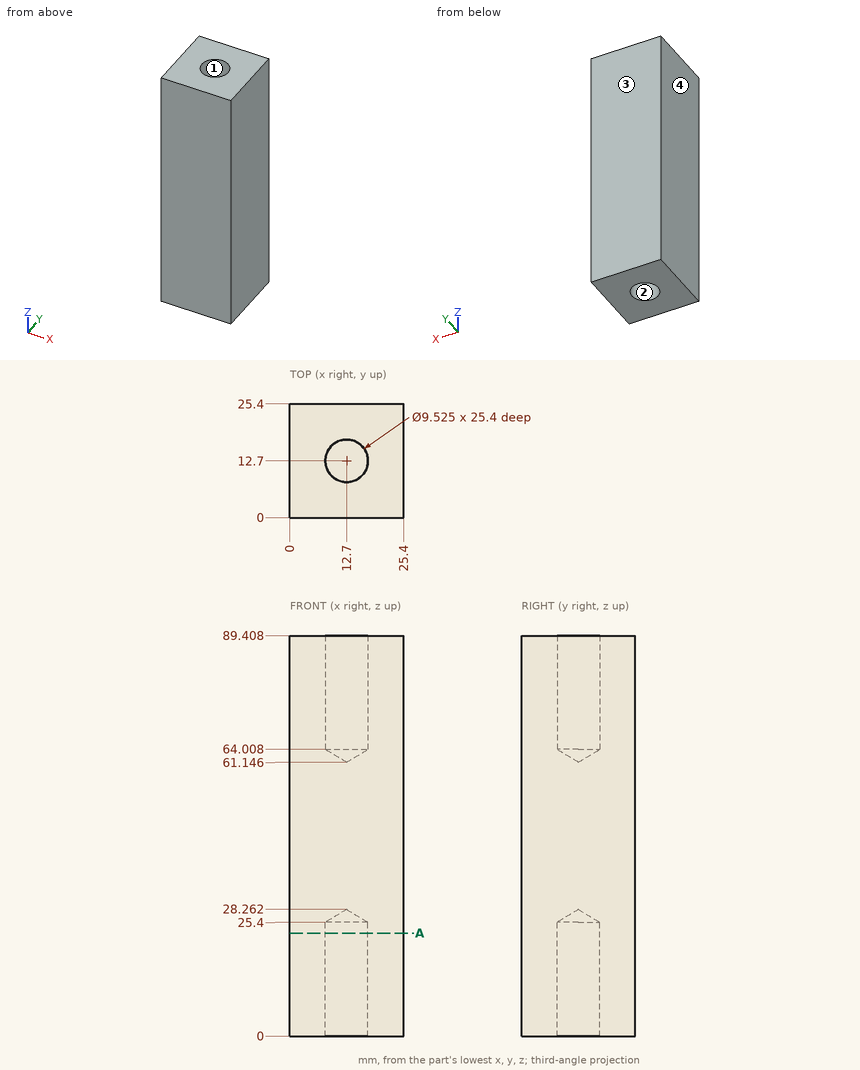
Study the drawing (mm; zero at the part's minimum x, y, z) and answer. Give positions to 0.01 mm unless a question says otherwise; leave off trailing zeros. Loops run counter-clockwise (first coordinate to the right, second up) from the corner with the lowest first, then second, coordinate; pieces in that order, holes last. Notation, with made-up numbers: (1.5, 65.25) - (33.5, 65.25) arc R30 cw to (33.5, 99.25) - close; hole circle Ø5 at (-37.5, -36.75). An arc over 180 degrees is marked (long way). Answer in a Markdown table with one row per item. Add a question column.
Q1. Determine the mould class of the marked faces 1, 2, 3 and 4 for opening direction Y: released by +Y, released by -Y, zero draft, split by the parting line, or undercut.
Q2. Consider line 1 along X through (y, z) = (12.7, 78.5); line 2 along Z through (x, y) = (13, 16). Determine where each line is inside the solid, lowest interval first.
Q3. Each of these flat-tipped pins is pushed along its axis until it touches: P1, Ø2, axis at x = 16, y = 12, coming from the +Z side (1 decimal); P2, Ø1.5, axis at x = 14, y = 12.5, coming from the -Z side. Where does it stop, or does it pass through?
Q4. The part is cut by section A-A (z = 23). Determine the outline of the cut face in (x, y) (1 decimal), and give its area (3 significant figures).
Solution:
| question | item | result |
|---|---|---|
| 1 | face 1 | undercut |
| 1 | face 2 | undercut |
| 1 | face 3 | released by +Y |
| 1 | face 4 | zero draft |
| 2 | line 1 | x = 0 to 7.94, 17.46 to 25.4 |
| 2 | line 2 | z = 26.27 to 63.14 |
| 3 | P1 | stops at z = 63.8 |
| 3 | P2 | stops at z = 27.02 |
| 4 | outline | (0, 0) - (25.4, 0) - (25.4, 25.4) - (0, 25.4) - close; hole circle Ø9.5 at (12.7, 12.7) |
| 4 | area | 574 mm² |
